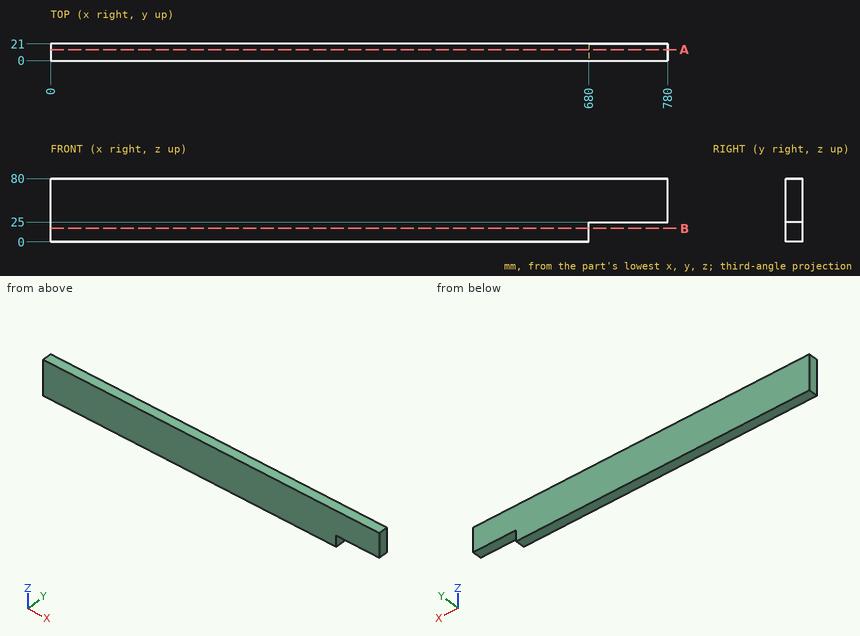
Job drawing, mm, ordinate dimensions from the low corner. One solid piece. Coordinates: 2 decimals unless noted, no trailing zeros. Order: outer loops, then holes, each group sorted by start corner. A loop starts at its lowest first (then second) coordinate and runs counter-clockwise, first axis right, second up. Notation, with made-up numbers: (39.5, -3) -> (75.5, -3) arc R18 ccw to (75.5, 19) -> close; hole circle Ø6 at (-9.75, 73). An arc over 180 degrees is marked (long way). Return JSON: item names as keys, results as strings. Group by question number.
Item 1: Saw through at A-A on y = 14. Write the cut outline in (x, z), then the cut area to 3 significant figures.
Item 2: Wall check: line 1 along Z through (x, y) = (735.5, 5.5); line 2 along X through (y, z) = (14.5, 4). Give the ranges that are in metal, low to high. Write a range as [from, to].
Item 3: Saw through at B-B on z = 17. Write the cut outline in (x, y), then the cut area to 3 significant figures.
Item 4: Flat gauge pin, fed straight in: P1, Ø10.5, axis at x = 718, y = 13, coming from the -Z side. Where does the tip first touch, or does it go through?
Values found:
{
 "1": {"outline": "(0, 0) -> (680, 0) -> (680, 25) -> (780, 25) -> (780, 80) -> (0, 80) -> close", "area": "59,900 mm2"},
 "2": {"line 1": "z = [25, 80]", "line 2": "x = [0, 680]"},
 "3": {"outline": "(0, 0) -> (680, 0) -> (680, 21) -> (0, 21) -> close", "area": "14,300 mm2"},
 "4": {"P1": "stops at z = 25"}
}
